Autodesk Inventor part; units mm, degrees
ref_plane "YZ Plane" through (0, 0, 0) normal (1, 0, 0) x (0, 1, 0)
ref_plane "XZ Plane" through (0, 0, 0) normal (0, 1, 0) x (-1, 0, 0)
ref_plane "XY Plane" through (0, 0, 0) normal (0, 0, 1) x (1, 0, 0)
sketch "Sketch1" plane through (0, 0, 0) normal (0, 0, 1) x (1, 0, 0)
  line L0 (717.55, 0) -> (717.55, 304.8)
  line L1 (717.55, 304.8) -> (0, 304.8)
  line L2 (0, 304.8) -> (0, 0)
  line L3 (250.825, 0) -> (250.825, 266.7)
  line L4 (250.825, 266.7) -> (466.725, 266.7)
  line L5 (466.725, 266.7) -> (466.725, 0)
  line L6 (466.725, 0) -> (717.55, 0)
  line L7 (250.825, 0) -> (0, 0)
  point P0 (358.775, 152.4)
  point P1 (358.775, 289.941)
  point P2 (239.661, 221.1705)
  point P3 (239.661, 83.6295)
  point P4 (358.775, 14.859)
  point P5 (477.889, 83.6295)
  point P6 (477.889, 221.1705)
  point P7 (12.7, 266.7)
  point P8 (12.7, 12.7)
  point P9 (704.85, 12.7)
  point P10 (704.85, 266.7)
  dimension "d0" = 717.55
  dimension "d1" = 304.8
  dimension "d2" = 358.775
  dimension "d3" = 152.4
  dimension "d4" = 137.541
  dimension "d7" = 360
  dimension "d11" = 38.1
  dimension "d21" = 38.1
  dimension "d22" = 12.7
  dimension "d23" = 12.7
  dimension "d24" = 12.7
  dimension "d25" = 12.7
  dimension "d26" = 12.7
  dimension "d27" = 12.7
  dimension "d28" = 38.1
  dimension "d36" = 107.95
  dimension "d37" = 107.95
extrude "Extrusion1" add sketch "Sketch1" against normal blind 3.175
hole "Hole1" at (358.775, 152.4, 0) at (358.775, 289.941, 0) at (239.661, 221.1705, 0) at (239.661, 83.6295, 0) at (358.775, 14.859, 0) at (477.889, 83.6295, 0) at (477.889, 221.1705, 0) direction (0, 0, -1) diameter 6.35 depth 25.4 tip angle 118
hole "Hole2" at (12.7, 266.7, 0) at (12.7, 12.7, 0) at (704.85, 12.7, 0) at (704.85, 266.7, 0) direction (0, 0, -1) diameter 6.35 depth 25.4 tip angle 118
properties part number "top plate"
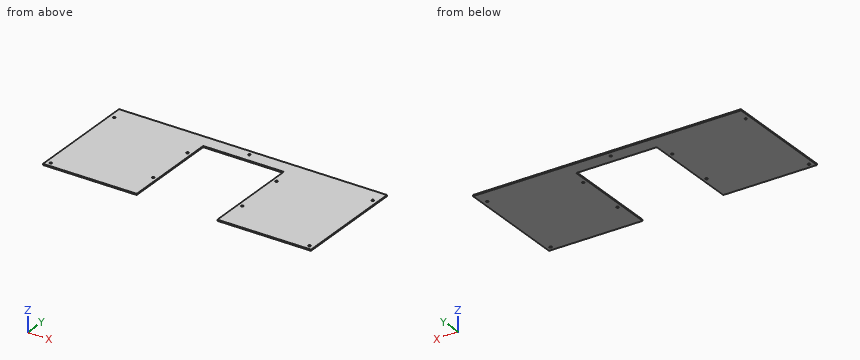
The listing builds one solid part. Answer for the finished solid, in the listing's coordinates (mm). Round coordinates to 2 decimals unless told otherwise and drop trailing zeros. Order: outer loops, then holes, each group sorted by start corner. A loop starts at its lowest first (then second) coordinate and runs counter-clockwise, first axis right, second up. Notation, with made-up numbers: (-32, -24) -> (4, -24) arc R5 cw to (4, -17) -> close; hole circle Ø4 at (89, -24). An arc over 180 degrees is marked (long way). One line per item, written item: value.
Item 1: Find section C-C, the plane x = 299.5. Give the vertices of the cut face in (y, z) (3 decimals), then the cut area to 3 significant figures.
Taken from the geometry:
outline: (266.7, -3.175) -> (304.8, -3.175) -> (304.8, 0) -> (266.7, 0) -> close
area: 121 mm2
Item 2: Find section A-A, the plane y = 252. Give the vertices of the cut face in (x, z) (3 decimals), then the cut area to 3 significant figures.
Taken from the geometry:
outline: (0, -3.175) -> (250.825, -3.175) -> (250.825, 0) -> (0, 0) -> close; (466.725, -3.175) -> (717.55, -3.175) -> (717.55, 0) -> (466.725, 0) -> close
area: 1,590 mm2
Item 3: Find section B-B, the plane z = -2.55. State how many separate pieces and enclosed holes the cut face has, then the cut area to 3 significant figures.
Taken from the geometry:
separate pieces: 1
enclosed holes: 9
area: 161,000 mm2
Item 4: Straight lines are drawn through the part: L1, parallel to Y at x = 12.7, z = -2.4 (3 decimals); L2, parallel to X at y = 12.7, z = -2.2 (3 decimals); L3, parallel to X at y = 18, z = -1.65 (3 decimals). For each, find the intervals that lie inside material, in ascending order.
Taken from the geometry:
L1: y = 0 to 9.525, 15.875 to 263.525, 269.875 to 304.8
L2: x = 0 to 9.525, 15.875 to 250.825, 466.725 to 701.675, 708.025 to 717.55
L3: x = 0 to 250.825, 466.725 to 717.55
